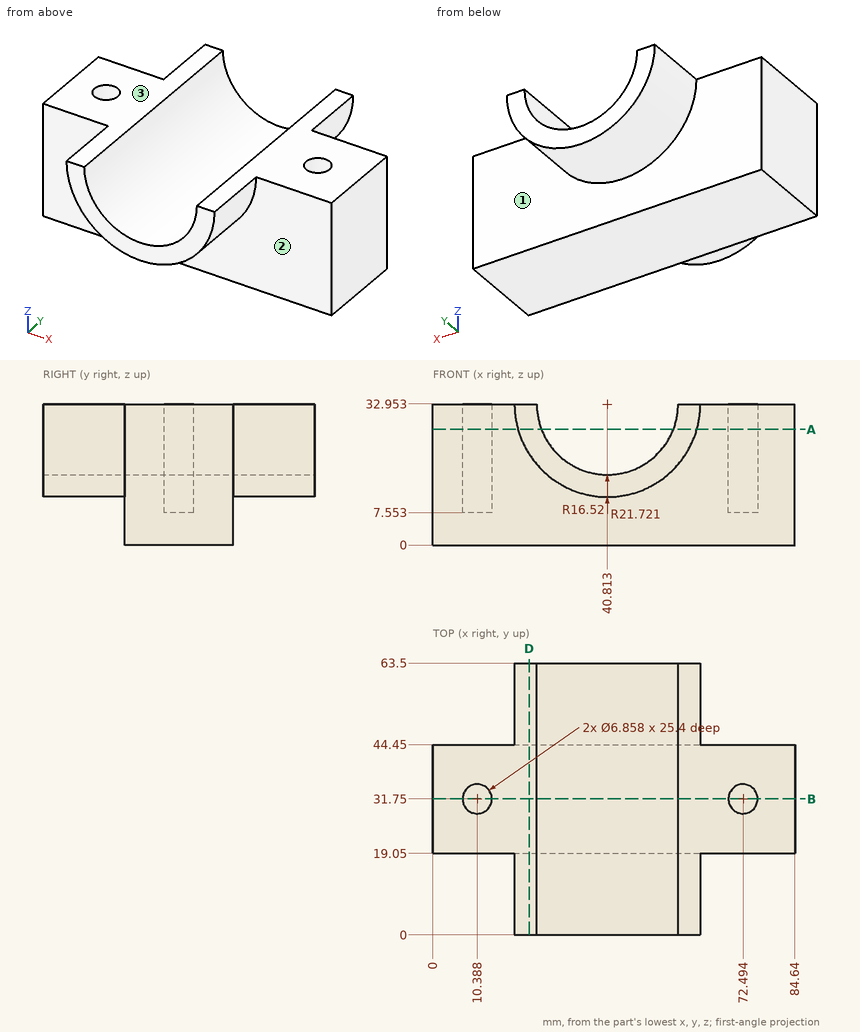
Check sheet for the drawn part. Datum: minimum x, y, z corner. Units: mm. A direction names the side the tool comes from. Round coordinates to 2 decimals unless told otherwise and drop trailing zeros. Order: outer loops, then holes, each group sorted by start corner. A loop starts at its lowest first (then second) coordinate and runs counter-clockwise, first axis right, second up.
(1) Go/stop test with flat-tipped pins: P1, Ø2, axis at x = 71, y = 33.5, coming from the +Z side; P2, Ø8, axis at x = 36, y = 7, coming from the -Z side; P3, Ø12, axis at y = 10, z = 19, coming from the +X side (1 decimal). Record where each tip stops, or that it passes through.
(2) Access from +Z, -Z, +X, -X, +Y, -Y to the whole of each face (thin tool, end or side, straight path). Record for the marked faces 1, 2 and 3.
(3) Scan lines: probe 1 along X at (y, z) = (31, 13) (1 decimal); probe 2 along X at (y, z) = (29, 24) (1 decimal); probe 3 along Y at (x, z) = (30.5, 9). Record each from-to range of solid material in increasing order.
(4) Cross-section at A-A, the plane z = 27. State how many separate pieces and enclosed holes the cut face has, and give its area (3 significant figures).
(5) Cross-section at D-D, the plane x = 22.5. Enter the section's corners in (y, z).
(6) Cross-section at B-B, the plane y = 31.75. Enter the section's corners in (x, z) (1 decimal).
Check sheet entries:
1. P1: stops at z = 7.55
1. P2: stops at z = 11.25
1. P3: stops at x = 61
2. face 1: -Z, +Y
2. face 2: -Z, -Y
2. face 3: +Z, +X, -X, +Y, -Y
3. probe 1: x = 0 to 7, 13.7 to 69.1, 75.8 to 84.6
3. probe 2: x = 0 to 8.3, 12.4 to 26.9, 54.7 to 70.4, 74.5 to 84.6
3. probe 3: y = 19.05 to 44.45
4. separate pieces: 2
4. enclosed holes: 2
4. area: 1,710 mm2
5. outline: (0, 21.27) - (19.05, 21.27) - (19.05, 0) - (44.45, 0) - (44.45, 21.27) - (63.5, 21.27) - (63.5, 32.95) - (0, 32.95) - close
6. outline: (0, 0) - (84.6, 0) - (84.6, 33) - (75.9, 33) - (75.9, 7.6) - (69.1, 7.6) - (69.1, 33) - (57.3, 33) arc R16.5 cw to (24.3, 33) - (13.8, 33) - (13.8, 7.6) - (7, 7.6) - (7, 33) - (0, 33) - close
